Could you check a few things on this drawing? It's one solid part, dimensions in mm from its lowest x, y, z. Round coordinates to 2 decimals unless told otherwise and drop trailing zeros. Write each loop counter-clockwise with the first axis right and the second up, starting at its lowest first coordinate (ties: lowest second). Pieces come first, ordered by that corner, then holes. Notation, with made-up numbers: M -37.75,-24 L -17.75,-24 A8 ccw -17.75,-11 Z; hole C 25,19.5 d1. An arc over 180 degrees is marked long. One line per question, with ' | ' between items. Start each with the question number.
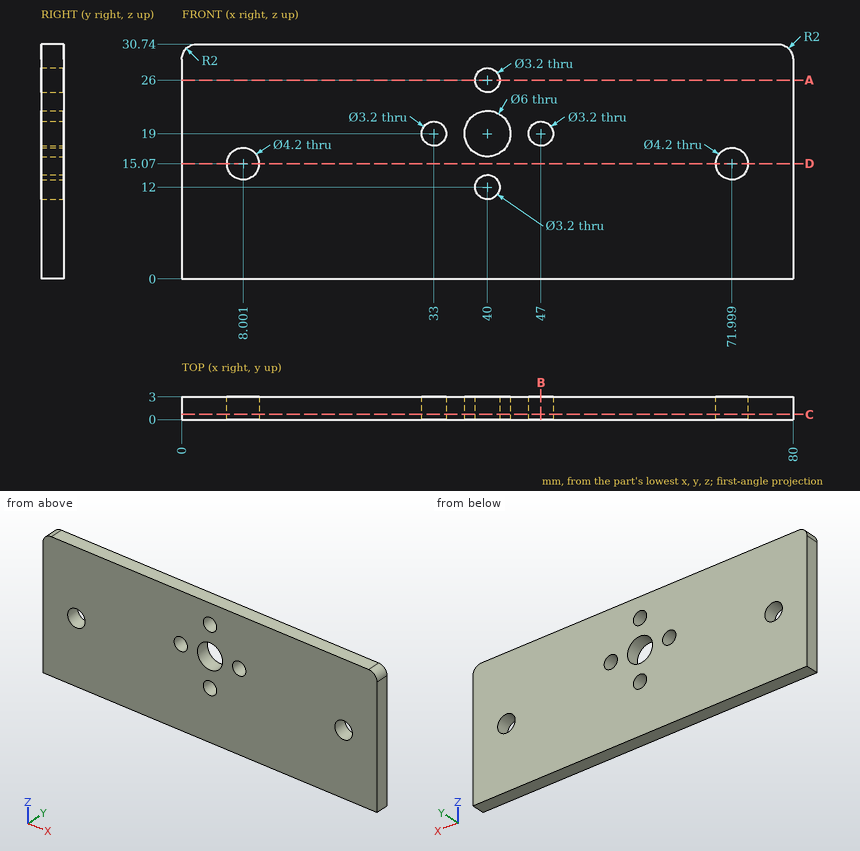
1. Suppose I cut it at A-A (z = 26). Write out the boundary of the cut face in (x, y), and give its area (3 significant figures).
2. I'm going to push a flat-ended pin straight in: P1, Ø1.9, axis at x = 33, z = 19, coming from the -Y side. Where does the tip first touch, or does it pass through?
3. Suppose I cut it at D-D (z = 15.07). Write out the boundary of the cut face in (x, y).
4. I need wall thicknesses on line 1 along X through (y, z) = (0.7, 15.07); line 2 along Z through (x, y) = (47, 2); line 3 along X through (y, z) = (2.45, 17). Which ranges of each line are inside material? Lowest first, please. Write a range as from..to.
5. Suppose I cut it at B-B (x = 47). Write out the boundary of the cut face in (y, z).
6. Suppose I cut it at C-C (y = 0.7). Write out the boundary of the cut face in (x, z), and give its area (3 significant figures).
Computed:
1) outline: M 0,0 L 38.4,0 L 38.4,3 L 0,3 Z; M 41.6,0 L 80,0 L 80,3 L 41.6,3 Z | area: 230 mm²
2) P1: passes through
3) outline: M 0,0 L 5.9,0 L 5.9,3 L 0,3 Z; M 10.1,0 L 69.9,0 L 69.9,3 L 10.1,3 Z; M 74.1,0 L 80,0 L 80,3 L 74.1,3 Z
4) line 1: x = 0..5.9, 10.1..69.9, 74.1..80 | line 2: z = 0..17.4, 20.6..30.74 | line 3: x = 0..7.17, 8.83..37.76, 42.24..71.17, 72.83..80
5) outline: M 0,0 L 3,0 L 3,17.4 L 0,17.4 Z; M 0,20.6 L 3,20.6 L 3,30.74 L 0,30.74 Z
6) outline: M 0,0 L 80,0 L 80,28.74 A2 ccw 78,30.74 L 2,30.74 A2 ccw 0,28.74 Z; hole C 8,15.07 d4.2; hole C 33,19 d3.2; hole C 40,19 d6; hole C 40,12 d3.2; hole C 40,26 d3.2; hole C 47,19 d3.2; hole C 72,15.07 d4.2 | area: 2,370 mm²
